Source: CAD feature listing. Evaluate the final solid. Frame: model axes, mm. Face numbers are marked on the shaded views. Give positions to 0.01 mm unless a question says otherwise; leave off trailing zeros. Order: outer loops, then holes, each group sorted by start corner. A loop starts at its lowest first (then second) coordinate and runs counter-clockwise, first axis right, second up. Notation, with made-up numbers: M 8.5,-15 L 65.5,-15 A13 ccw 65.5,-6 Z; hole C 86.25,76 d8. An arc over 180 degrees is marked long. Answer as a JSON object with one key per item and string values. Group by question number.
1. Section query A-A (y = 0). Output: boundary loops of the cut face in (x, z).
2. Pin query (flat end, axial travel): P1, Ø1, axis at y = 5.5, z = 2, coming from the -X side. Return the tip coordinate at first contact, or that it passes through.
3. Material intervals for L1, parallel to Y at x = 0, z = 4.15; L2, parallel to Y at x = 1.25, z = 0.95; L3, parallel to X at y = 0.75, z = 4.35, sorted ascending. Write a range as [from, to].
4. Section query C-C (z = 0.5). Output: boundary loops of the cut face in (x, y), plus the area to 3 significant figures.
5. Pull-direction query (Y, two-part tool) for the marked faces 1, 2 and 3; classes: +Y half, -Y half, draft (parallel to the pull), parting line (faces both ways), or undercut.
from build123d import *

# Parameters (mm, degrees)
SKETCH1_R           = 7.5
BOSS_EXTRUDE1_DEPTH = 6
SKETCH2_R           = 3
CUT_EXTRUDE1_DEPTH  = 6
FILLET1_R           = 0.2


with BuildPart() as part:
    # Sketch1 → Boss-Extrude1 (new body)
    with BuildSketch(Plane.XY):
        Circle(SKETCH1_R)
    extrude(amount=BOSS_EXTRUDE1_DEPTH)

    # Sketch2 → Cut-Extrude1 (cut)
    with BuildSketch(Plane.XY):
        with Locations(Location((0, 0, 0), (0, 0, 180))):
            Circle(SKETCH2_R)
    extrude(amount=CUT_EXTRUDE1_DEPTH, mode=Mode.SUBTRACT)

    # Fillet1
    fillet1_edges = [part.edges().sort_by_distance(p)[0] for p in [
        (-7.5, 0, 0),
        (-7.5, 0, 6),
    ]]
    fillet(fillet1_edges, radius=FILLET1_R)


solid = part.part
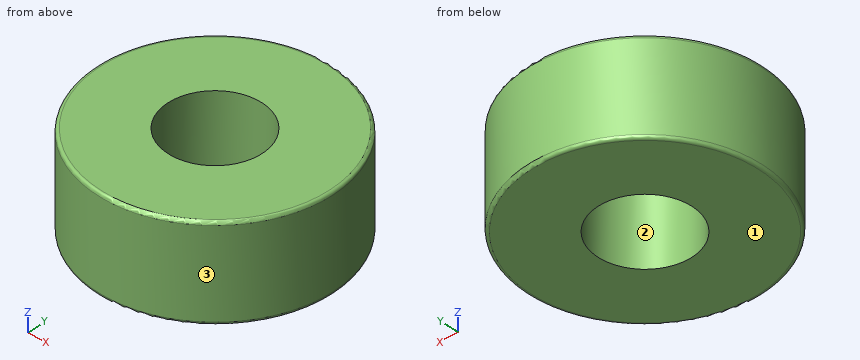
Answer sheet:
{
 "1": {"outline": "M -7.5,0.2 A0.2 ccw -7.3,0 L -3,0 L -3,6 L -7.3,6 A0.2 ccw -7.5,5.8 Z; M 3,0 L 7.3,0 A0.2 ccw 7.5,0.2 L 7.5,5.8 A0.2 ccw 7.3,6 L 3,6 Z"},
 "2": {"P1": "x = -5.59"},
 "3": {"L1": "[-7.5, -3], [3, 7.5]", "L2": "[-7.4, -2.73], [2.73, 7.4]", "L3": "[-7.46, -2.9], [2.9, 7.46]"},
 "4": {"outline": "C 0,0 d15; hole C 0,0 d6", "area": "148 mm^2"},
 "5": {"face 1": "draft", "face 2": "undercut", "face 3": "parting line"}
}
